from build123d import *

# Parameters (mm, degrees)
F0_W     = 10
F0_H     = 10
F1_DEPTH = 35
F2_R     = 1.5
F3_DEPTH = 12


with BuildPart() as f1:
    # F0 (on Front) → F1 (new body)
    with BuildSketch(Plane.XZ):
        with Locations((-5, 5)):
            Rectangle(F0_W, F0_H)
    extrude(amount=F1_DEPTH)

    # F2 (on face) → F3 (cut)
    with BuildSketch(Plane.YZ):
        with Locations((-28.746059, 5)):
            Circle(F2_R)
        with Locations((-13.746059, 4.852584)):
            Circle(F2_R)
    extrude(amount=-F3_DEPTH, mode=Mode.SUBTRACT)


solid = f1.part
Geometry check sheet. Reference: the model listing, model coordinates, mm. Round coordinates to 2 decimals unless told otherwise and drop trailing zeros. Loops run counter-clockwise (first coordinate to the right, second up) from the corner with the lowest first, then second, coordinate; pieces in that order, holes last.
Item 1: Cross-section at B-B on y = -13.5. Record the boundary of the cut face in (x, z).
Item 2: Thickness scan on line 1 (Y direction, x = -7, z = 5.25); line 2 (Y direction, x = -6, z = 6); line 3 (Z direction, x = -8.5, y = -28). Record the ranges inside material, lowest first.
Item 3: Cross-section at D-D on z = 4. Record the boundary of the cut face in (x, y).
Item 4: Cross-section at C-C on x = -2.25. Record the boundary of the cut face in (y, z).
Item 5: Mould release check, pull along Z, two halves, no side actions. Record for faces 1 (the flat face through (-5, -17, 0)), 2 (the cylindrical face through (-4.93, -12.315, 5.303)), 3 (the flat face through (-10, -17, 5)): pulls with the +Z half, pulls with the -Z half, needs draft (parallel to the pull), parting line crosses it, or undercut.
Item 6: Cross-section at A-A on z = 6. Record the boundary of the cut face in (x, y), then the cut area to 3 significant figures.
Answer sheet:
1. outline: (-10, 0) - (0, 0) - (0, 3.37) - (-10, 3.37) - close; (-10, 6.33) - (0, 6.33) - (0, 10) - (-10, 10) - close
2. line 1: y = -35 to -30.23, -27.27 to -15.19, -12.3 to 0
2. line 2: y = -35 to -29.86, -27.63 to -14.71, -12.78 to 0
2. line 3: z = 0 to 3.7, 6.3 to 10
3. outline: (-10, -35) - (0, -35) - (0, -29.86) - (-10, -29.86) - close; (-10, -27.63) - (0, -27.63) - (0, -14.98) - (-10, -14.98) - close; (-10, -12.51) - (0, -12.51) - (0, 0) - (-10, 0) - close
4. outline: (-35, 0) - (0, 0) - (0, 10) - (-35, 10) - close; hole circle Ø3 at (-28.75, 5); hole circle Ø3 at (-13.75, 4.85)
5. face 1: pulls with the -Z half
5. face 2: undercut
5. face 3: needs draft
6. outline: (-10, -35) - (0, -35) - (0, -29.86) - (-10, -29.86) - close; (-10, -27.63) - (0, -27.63) - (0, -14.71) - (-10, -14.71) - close; (-10, -12.78) - (0, -12.78) - (0, 0) - (-10, 0) - close
6. area: 308 mm2
